Check sheet for the drawn part. Datum: minimum x, y, z corner. Units: mm. Give positions to 0.01 mm unless a question says otherwise; leave off trailing zeros. Loops run counter-clockwise (first coordinate to the right, second up) from the corner with the lowest first, then second, coordinate; pieces in that order, holes last. Notation, with made-up numbers: (54, 26.25) - (98, 26.25) arc R18 ccw to (98, 32.25) - close; hole circle Ø8 at (-34.5, -7.75). An arc over 180 degrees is marked (long way). One line per item, written item: value. Start each with the question number.
1. Sectioned sample at D-D (y = 145). Record the cut outline in (x, z) (1 decimal), plus the area to 3 significant figures.
2. Sectioned sample at B-B (x = 25). Record the cut outline in (y, z) (1 decimal), plus the area to 3 significant figures.
3. Mould release check, pull along Z, two halves, no side actions. Record for the marked faces 1, 2, 3 and 4: pulls with the +Z half, pulls with the -Z half, needs draft (parallel to the pull), parting line crosses it, or undercut.
4. Sectioned sample at A-A (z = 35). Record the cut outline in (x, y).
5. Gauge pin test, flat ends, axial feed: pin 1 (5 mm diameter, centred on x = 101, z = 28, fed in from -Y); pin 2 (23.5 mm diameter, centred on x = 145, z = 35, fed in from +Y); pin 3 (12 mm diameter, centred on y = 102.5, z = 36, fed in from -X); pin 4 (8 mm diameter, centred on y = 89, z = 61.5, fed in from -X). Record the tip position at first contact, or that the pin passes through.
6. Sectioned sample at C-C (y = 174). Record the cut outline in (x, z).
7. Scan lines: L1, parallel to Z at x = 196.75, y = 25; L2, parallel to Z at x = 177.5, y = 78.5; L3, parallel to X at y = 100.5, z = 31. Record each from-to range of solid material in increasing order. Write a range as [from, to].
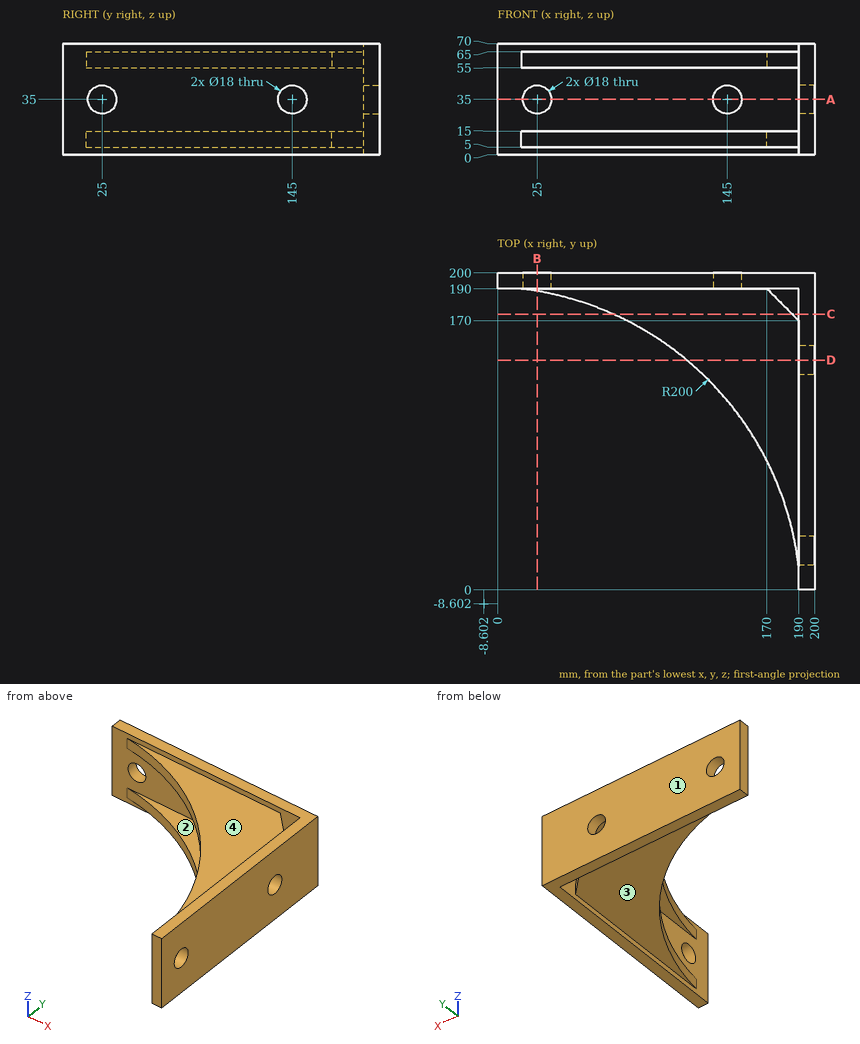
Results are:
1. outline: (119.5, 5) - (190, 5) - (190, 0) - (200, 0) - (200, 26) - (190, 26) - (190, 15) - (119.5, 15) - close; (119.5, 55) - (190, 55) - (190, 44) - (200, 44) - (200, 70) - (190, 70) - (190, 65) - (119.5, 65) - close
1. area: 1,930 mm^2
2. outline: (188.6, 5) - (190, 5) - (190, 0) - (200, 0) - (200, 26) - (190, 26) - (190, 15) - (188.6, 15) - close; (188.6, 55) - (190, 55) - (190, 44) - (200, 44) - (200, 70) - (190, 70) - (190, 65) - (188.6, 65) - close
2. area: 549 mm^2
3. face 1: needs draft
3. face 2: undercut
3. face 3: pulls with the -Z half
3. face 4: pulls with the +Z half
4. outline: (0, 190) - (16, 190) - (16, 200) - (0, 200) - close; (34, 190) - (136, 190) - (136, 200) - (34, 200) - close; (154, 190) - (190, 190) - (190, 154) - (200, 154) - (200, 200) - (154, 200) - close; (190, 0) - (200, 0) - (200, 16) - (190, 16) - close; (190, 34) - (200, 34) - (200, 136) - (190, 136) - close
5. pin 1: stops at y = 190
5. pin 2: stops at y = 200
5. pin 3: stops at x = 190
5. pin 4: stops at x = 163.67
6. outline: (72.98, 5) - (186, 5) - (186, 15) - (72.98, 15) - close; (72.98, 55) - (186, 55) - (186, 65) - (72.98, 65) - close; (190, 0) - (200, 0) - (200, 70) - (190, 70) - close
7. L1: z = [0, 26], [44, 70]
7. L2: z = [5, 15], [55, 65]
7. L3: x = [190, 200]
